```python
from build123d import *

# Parameters (mm, degrees)
F1_DEPTH = 6.35
F2_R     = 3.81
F3_R     = 1.27


with BuildPart() as f1:
    # F0 (on Top) → F1 (new body)
    with BuildSketch(Plane.XY):
        with BuildLine():
            Line((45.085, -62.865), (45.085, 0))
            ThreePointArc((45.085, 0), (0, 45.085), (-45.085, 0))
            Line((-45.085, 0), (-45.085, -62.865))
            Line((-45.085, -62.865), (-38.735, -62.865))
            Line((-38.735, -62.865), (-38.735, -37.465))
            Line((-38.735, -37.465), (-33.02, -37.465))
            Line((-33.02, -37.465), (-33.02, 0))
            ThreePointArc((-33.02, 0), (0, 33.02), (33.02, 0))
            Line((33.02, 0), (33.02, -37.465))
            Line((33.02, -37.465), (38.735, -37.465))
            Line((38.735, -37.465), (38.735, -62.865))
            Line((38.735, -62.865), (45.085, -62.865))
        make_face()
    extrude(amount=F1_DEPTH)

    # F2
    f2_edges = [f1.edges().sort_by_distance(p)[0] for p in [
        (-45.085, -62.865, 3.175),
        (45.085, -62.865, 3.175),
    ]]
    fillet(f2_edges, radius=F2_R)

    # F3
    f3_edges = [f1.edges().sort_by_distance(p)[0] for p in [
        (-38.735, -62.865, 3.175),
        (38.735, -62.865, 3.175),
    ]]
    fillet(f3_edges, radius=F3_R)


solid = f1.part
```
Design review of the part built by this model. Coordinates are the model's own, in mm. A direction names the side the tool comes from. Give positions to 0.01 mm unless a question says otherwise; leave off trailing zeros. Write each loop counter-clockwise with the first axis right and the second up, starting at its lowest first coordinate (ties: lowest second). Pieces come first, ordered by that corner, then holes.
(1) Mouldability with a two-part tool opening along X and no side actions: class faces 3 (the face through (38.735, -49, 3)), 4 (the face through (-44, -61.72, 3.22)), 5 (the face through (-34, -5, 6.35)) as +X half, -X half, draft (parallel to the pull), parting line (faces both ways), or undercut.
Checked values:
face 3: undercut
face 4: -X half
face 5: draft
(2) Wall thickness on line 1 along X through (y, z) = (-54.5, 2.75) (3 decimals); line 2 along X through (y, z) = (-28, 2) (3 decimals); line 3 along Y through (x, z) = (-25.5, 4.5): over which ranges is each line inside the solid? List them lowest first.
Checked values:
line 1: x = -45.085 to -38.735, 38.735 to 45.085
line 2: x = -45.085 to -33.02, 33.02 to 45.085
line 3: y = 20.98 to 37.18
(3) Tool access review of faces 1 (the face through (33.02, -18, 3)), 2 (the face through (0.991, 45.074, 3.131)): name each direction out of +Z, -Z, +X, -X, +Y, -Y from which nothing blocks a thin tool from reaching the whole face with its end or side.
Checked values:
face 1: +Z, -Z, -Y
face 2: +Z, -Z, +Y
(4) Add section A-A (y = -6). Give the boundary of the cut face in (x, z) (3 decimals).
Checked values:
outline: (-45.085, 0) - (-33.02, 0) - (-33.02, 6.35) - (-45.085, 6.35) - close; (33.02, 0) - (45.085, 0) - (45.085, 6.35) - (33.02, 6.35) - close
(5) Add section D-D (x = 0). Give the boundary of the cut face in (y, z) (3 decimals).
Checked values:
outline: (33.02, 0) - (45.085, 0) - (45.085, 6.35) - (33.02, 6.35) - close
(6) Add section C-C (z = 2). Give the boundary of the cut face in (x, y) (3 decimals), and give its area (3 significant figures).
Checked values:
outline: (-45.085, -59.055) arc R3.81 ccw to (-41.275, -62.865) - (-40.005, -62.865) arc R1.27 ccw to (-38.735, -61.595) - (-38.735, -37.465) - (-33.02, -37.465) - (-33.02, 0) arc R33.02 cw to (33.02, 0) - (33.02, -37.465) - (38.735, -37.465) - (38.735, -61.595) arc R1.27 ccw to (40.005, -62.865) - (41.275, -62.865) arc R3.81 ccw to (45.085, -59.055) - (45.085, 0) arc R45.085 ccw to (-45.085, 0) - close
area: 2,700 mm2
(7) Add section B-B (y = -40.5). Give the boundary of the cut face in (x, z) (3 decimals).
Checked values:
outline: (-45.085, 0) - (-38.735, 0) - (-38.735, 6.35) - (-45.085, 6.35) - close; (38.735, 0) - (45.085, 0) - (45.085, 6.35) - (38.735, 6.35) - close
(8) Clearance check with flat-ended pins moving along their axes: pin 1 Ø1.7 at (x, z) = (-35.5, 2) entering from -Y (3 decimals); pin 2 Ø1.5 at (y, z) = (12.5, 0.5) entering from +X; pin 3 Ø3 at (x, z) = (7, 3.5) entering from -Y. State where each tip first meets the part, or that it passes through.
Checked values:
pin 1: stops at y = -37.465
pin 2: stops at x = 43.53
pin 3: stops at y = 31.91
